Geometry check sheet. Reference: the model listing, model coordinates, mm. Face numbers are marked on the shaded views. A direction names the side the tool comes from. Coordinates: 2 decimals unless noted, no trailing zeros. Write each loop counter-clockwise with the first axis right and the second up, starting at its lowest first coordinate (ties: lowest second). Pieces come first, ordered by that corner, then holes. Notation, with made-up numbers: (10, -22) -> (49, -22) arc R10 ccw to (49, -9) -> close; hole circle Ø4 at (76.5, 80.25). An arc over 180 degrees is marked (long way). Use a Markdown table: item, result.
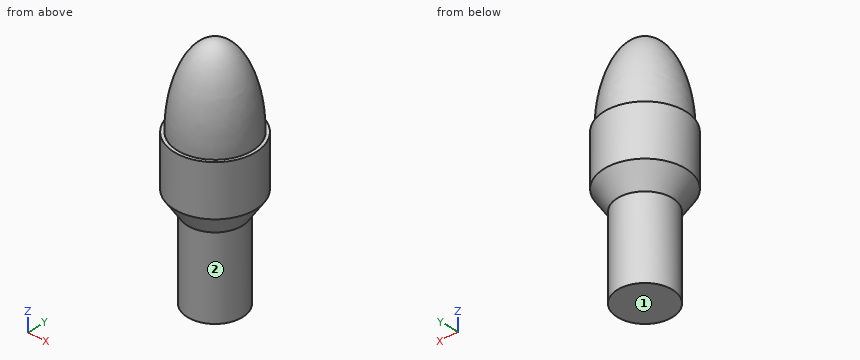
```python
from build123d import *

# Parameters (mm, degrees)
F0_R      = 13.5
F1_DEPTH  = 40
F1_FACE_R = 13.5
F2_DEPTH  = 10
F2_TAPER  = -33.02
F3_DEPTH  = 25


with BuildPart() as f1:
    # F0 (on Top) → F1 (new body)
    with BuildSketch(Plane.XY):
        Circle(F0_R)
    extrude(amount=F1_DEPTH)

    # F1_face (on face) → F2 (join)
    with BuildSketch(Plane.XY.offset(40)):
        Circle(F1_FACE_R)
    extrude(amount=F2_DEPTH, taper=F2_TAPER)

    # F3 (add): a face of the model
    f3_faces = [f1.faces().sort_by_distance(p)[0] for p in [
        (0, 0, 50),
    ]]
    extrude(f3_faces, amount=F3_DEPTH)

    # F4 (on Right) → F5 (revolve)
    with BuildSketch(Plane.YZ):
        with BuildLine():
            add(Edge.make_bspline(
                [(0, 115), (-18.4366899531, 115), (-18.4366899531, 75.3298997879), (-18.4366899531, 35.6597995758), (0, 35.6597995758)],
                knots=[0, 0, 0, 1.5707963268, 1.5707963268, 3.1415926536, 3.1415926536, 3.1415926536], degree=2, weights=[1, 0.7071067812, 1, 0.7071067812, 1]))
            Line((0, 35.6597995758), (0, 115))
        make_face()
    revolve(axis=Axis((0, 0, 57.5), (0, 0, 1)))


solid = f1.part
```
Item 1: Section check A-A on z = 66. Record the boundary of the cut face in (x, y), then the cut area to 3 significant figures.
Answer block:
| item | result |
|---|---|
| outline | circle Ø40 at (0, 0) |
| area | 1,260 mm^2 |
Item 2: Thickness scan on L1, parallel to Y at x = 0, z = 31; L2, parallel to Y at x = 4, z = 81; L3, parallel to Z at x = -1, y = 7. Record the ranges inside material, lowest first. Write a range as [from, to].
Answer block:
| item | result |
|---|---|
| L1 | y = [-13.5, 13.5] |
| L2 | y = [-17.8, 17.8] |
| L3 | z = [0, 111.97] |
Item 3: Tool access check on the marked faces 1 and 2. Record the directions out of +Z, -Z, +X, -X, +Y, -Y that give a thin tool (end or side, any length) a straight path to the whole face; none if there is none.
Answer block:
| item | result |
|---|---|
| face 1 | -Z, +X, -X, +Y, -Y |
| face 2 | -Z |
Item 4: Section check B-B on z = 44. Record the boundary of the cut face in (x, y), then the cut area to 3 significant figures.
Answer block:
| item | result |
|---|---|
| outline | circle Ø32.2 at (0, 0) |
| area | 814 mm^2 |
Item 5: Depth check by flat-ended pin: P1, Ø12, axis at x = 9.5, y = -1.5, coming from the +Z side; P2, Ø12, axis at x = 14.5, y = 9.5, coming from the +Z side; P3, Ø1.5, axis at x = 1, z = 13, coming from the -Y side. Enter the tip coordinate at first touch or a pass-through.
Answer block:
| item | result |
|---|---|
| P1 | stops at z = 114.23 |
| P2 | stops at z = 106.62 |
| P3 | stops at y = -13.5 |
